```python
from build123d import *

# Parameters (mm, degrees)
F1_DEPTH = 25.4
F3_D     = 9.525
F4_R     = 6.35


with BuildPart() as f1:
    # F0 (on Front) → F1 (new body)
    with BuildSketch(Plane.XZ):
        Polygon((0, 0), (-19.05, 0), (-19.05, -12.7), (12.7, -12.7), (12.7, 0), (12.7, 12.7), (0, 12.7), align=None)
    extrude(amount=-F1_DEPTH)

    # F3 (through all)
    with Locations(Plane.XY):
        with Locations((-9.525, 12.7)):
            Hole(F3_D / 2)

    # F4
    f4_edges = [f1.edges().sort_by_distance(p)[0] for p in [
        (-19.05, 25.4, -6.35),
        (-19.05, 0, -6.35),
    ]]
    fillet(f4_edges, radius=F4_R)

    # F5: F1 across face


with BuildPart() as f1_1:
    add(f1.part)
    add(f1.part.mirror(Plane(origin=(12.7, 12.7, 0), x_dir=(0, 1, 0), z_dir=(1, 0, 0))))


solid = f1_1.part
```
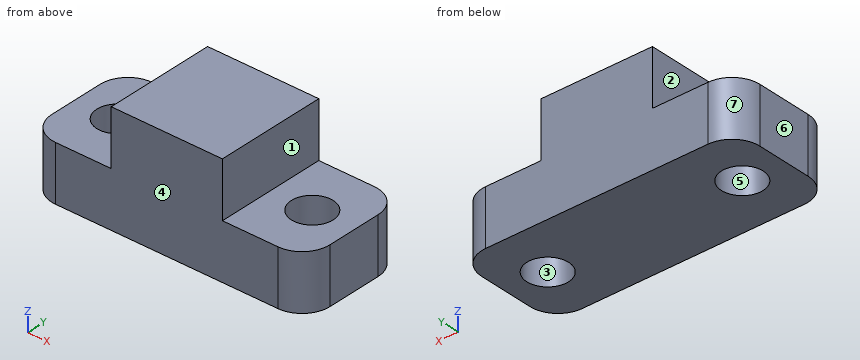
CAD build for the part. Positions are in the model's coordinates, mm. Face numbers are marked on the shaded views. A direction names the side the tool comes from. Round coordinates to 2 decimals unless told otherwise and drop trailing zeros. Loops run counter-clockwise (first coordinate to the right, second up) from the corner with the lowest first, then second, coordinate; pieces in that order, holes last. Notation, with made-up numbers: (53, -31) - (108, -31) arc R21 ccw to (108, 7) - close; hole circle Ø3 at (60, 1.5). An arc over 180 degrees is marked (long way). Return JSON: item names as keys, results as strings. Group by question number.
Q1. Drill centre lines: line 1 along X through (y, z) = (12, -1.75); line 2 along X through (y, z) = (15.75, -8.5); line 3 along X through (y, z) = (20.5, 9.25). Where is each one in solid material? Low to high. Write a range as [from, to].
Q2. Two-plate mould, pull along Y, no slides. Class the marked faces 4, 5, 6 and 7: +Y half, -Y half, draft (parallel to the pull), parting line (faces both ways), or undercut.
Q3. Band-saw the part on D-D on y = 19.75. Give the cut face in (x, z).
Q4. Band-saw the part on C-C on x = -9. Give the cut face in (y, z).
Q5. Band-saw the part on B-B on z = -0.75. Give the number of separate pieces and of enclosed holes in the cut face, plus the area to 3 significant figures.
Q6. Flat gauge pins, fed straight in: pin 1 Ø15 at (x, y) = (-12, 13.5) entering from +Z; pin 2 Ø7.5 at (x, y) = (-9.525, 12.7) entering from -Z; pin 3 Ø2 at (y, z) = (21.5, -5) entering from -X; pin 4 Ø14 at (y, z) = (19, 7.5) entering from -X. Where does each tip first touch, or does it go through?
Q7. Tool access for the marked faces 1, 2 and 3: list every direction of +Z, -Z, +X, -X, +Y, -Y with a clear straight run to the whole face (end or side of a thin tool).
Q8. Band-saw the part on A-A on y = 12.7. Give the cut face in (x, z).
Solutions:
{
 "1": {"line 1": "x = [-19.05, -14.24], [-4.81, 30.21], [39.64, 44.45]", "line 2": "x = [-19.05, -13.18], [-5.87, 31.27], [38.58, 44.45]", "line 3": "x = [0, 25.4]"},
 "2": {"face 4": "-Y half", "face 5": "undercut", "face 6": "draft", "face 7": "+Y half"},
 "3": {"outline": "(-19.01, -12.7) - (44.41, -12.7) - (44.41, 0) - (25.4, 0) - (25.4, 12.7) - (0, 12.7) - (0, 0) - (-19.01, 0) - close"},
 "4": {"outline": "(0, -12.7) - (7.97, -12.7) - (7.97, 0) - (0, 0) - close; (17.43, -12.7) - (25.4, -12.7) - (25.4, 0) - (17.43, 0) - close"},
 "5": {"separate pieces": "1", "enclosed holes": "2", "area": "1,440 mm^2"},
 "6": {"pin 1": "stops at z = 0", "pin 2": "passes through", "pin 3": "stops at x = -18.88", "pin 4": "stops at x = 0"},
 "7": {"face 1": "+Z, +X, +Y, -Y", "face 2": "+Z, -X, +Y, -Y", "face 3": "+Z, -Z"},
 "8": {"outline": "(-19.05, -12.7) - (-14.29, -12.7) - (-14.29, 0) - (-19.05, 0) - close; (-4.76, -12.7) - (30.16, -12.7) - (30.16, 0) - (25.4, 0) - (25.4, 12.7) - (0, 12.7) - (0, 0) - (-4.76, 0) - close; (39.69, -12.7) - (44.45, -12.7) - (44.45, 0) - (39.69, 0) - close"}
}
